```python
from build123d import *

# Parameters (mm, degrees)
SKETCH1_W           = 318
SKETCH1_H           = 8
BOSS_EXTRUDE1_DEPTH = 4.8
BOSS_EXTRUDE2_DEPTH = 0.79375
BOSS_EXTRUDE3_DEPTH = 0.79375
BOSS_EXTRUDE4_DEPTH = 0.79375
FILLET1_R           = 2.5


with BuildPart() as part:
    # Sketch1 → Boss-Extrude1 (new, symmetric)
    with BuildSketch(Plane.XY):
        Rectangle(SKETCH1_W, SKETCH1_H)
    extrude(amount=BOSS_EXTRUDE1_DEPTH, both=True)

    # Sketch3 → Boss-Extrude2 (add, symmetric)
    with BuildSketch(Plane.XY):
        Polygon((-64, 0), (-46.939710612, 195), (16.260289388, 195), (16, 0), align=None)
    boss_extrude2 = extrude(amount=BOSS_EXTRUDE2_DEPTH, both=True)

    # Mirror1: Boss-Extrude2 across plane
    add(boss_extrude2.mirror(Plane.ZX))

    # Sketch6 → Boss-Extrude3 (add, symmetric)
    with BuildSketch(Plane(origin=(0, 0, 0), x_dir=(1, 0, 0), z_dir=(0, 1, 0))):
        Polygon((159, -4.8), (166.766007972, -74.8), (145.966007972, -74.8), (107, -4.8), align=None)
    extrude(amount=BOSS_EXTRUDE3_DEPTH, both=True)

    # Sketch8 → Boss-Extrude4 (add, symmetric)
    with BuildSketch(Plane.XY):
        Polygon((159, 0), (177.834948036, 85.2), (153.758948036, 85.2), (112.7, 0), align=None)
    boss_extrude4 = extrude(amount=BOSS_EXTRUDE4_DEPTH, both=True)

    # Mirror2: Boss-Extrude4 across plane
    add(boss_extrude4.mirror(Plane.ZX))

    # Fillet1
    fillet1_edges = [part.edges().sort_by_distance(p)[0] for p in [
        (-159, 0, 4.8),
        (-159, 0, -4.8),
    ]]
    fillet(fillet1_edges, radius=FILLET1_R)


solid = part.part
```
Could you check a few things on this model? Use its own coordinates, in mm. A direction names the side the tool comes from. Round coordinates to 2 decimals unless told otherwise and drop trailing zeros. Write each loop counter-clockwise with the first axis right and the second up, starting at its lowest first coordinate (ties: lowest second). Pieces come first, ordered by that corner, then holes. Notation, with made-up numbers: M -11,32.5 L 5,32.5 A17 cw 5,36.5 Z; hole C 21,2.5 d9. An arc over 180 degrees is marked long. Answer in a Markdown table with one row per item. Add a question column.
Q1. Will these pins go through, and if not, where does the flat tip stop? pin 1 Ø24 at (x, y) = (-13.5, -86.5) entering from +Z; pin 2 Ø5 at (x, z) = (-28, 2) entering from +Y; pin 3 Ø19 at (x, y) = (132, -60.5) entering from -Z; pin 4 Ø8 at (x, z) = (103, 5) entering from +Y.
Q2. Imagine slicing it at C-C (z = 66.5). Please give me the cut outline in (x, y).
Q3. Imagine slicing it at A-A (y = 27). Please give me the cut outline in (x, z), then the cut area to 3 significant figures.
Q4. If I drill on line 1 (Y direction, x = 145, z = 32); line 2 (X direction, y = -1, z = 2), over which ranges is the centre line in solid material (lowest first)? Write a range as from..to.
Q5. Imagine slicing it at D-D (y = -23.5). Please give me the cut outline in (x, z).
Q6. If we mould it in two halves opening along X, with no side actions, what happens to faces 1 (the flat face through (134.47, 45.17, 0.01)), 2 (the flat face through (168.286, -42.004, 0.011)), 3 (the flat face through (-23, 101, -0.794))? For each: +X half, -X half, draft (parallel to the pull), parting line (faces both ways), or undercut.
Q7. Imagine slicing it at B-B (x = -19). Please give me the cut outline in (y, z), then the cut area to 3 significant figures.
Q8. On a 3-axis mill with a long thin cutter (end or side, diameter ignored), from which of +Z, -Z, +X, -X, +Y, -Y can I reach the whole of each face in a straight line? I mean faces 4 (the flat face through (-55.412, -98.163, 0.011)), 5 (the flat face through (144, -0.794, 32)), 6 (the flat face through (134.47, -45.17, 0.01)), 7 (the flat face through (-23, 101, 0.794)), 8 (the flat face through (-23, -101, -0.794)). Say none if no direction works.
Values:
| question | item | result |
|---|---|---|
| 1 | pin 1 | z = 0.79 |
| 1 | pin 2 | y = 195 |
| 1 | pin 3 | z = -0.79 |
| 1 | pin 4 | y = 4 |
| 2 | outline | M 141.35,-0.79 L 165.85,-0.79 L 165.85,0.79 L 141.35,0.79 Z |
| 3 | outline | M -61.64,-0.79 L 16.04,-0.79 L 16.04,0.79 L -61.64,0.79 Z; M 125.71,-0.79 L 164.97,-0.79 L 164.97,0.79 L 125.71,0.79 Z |
| 3 | area | 186 mm^2 |
| 4 | line 1 | -0.79..0.79 |
| 4 | line 2 | -159..159 |
| 5 | outline | M -61.94,-0.79 L 16.03,-0.79 L 16.03,0.79 L -61.94,0.79 Z; M 124.02,-0.79 L 164.2,-0.79 L 164.2,0.79 L 124.02,0.79 Z |
| 6 | face 1 | undercut |
| 6 | face 2 | +X half |
| 6 | face 3 | draft |
| 7 | outline | M -195,-0.79 L -4,-0.79 L -4,-4.8 L 4,-4.8 L 4,-0.79 L 195,-0.79 L 195,0.79 L 4,0.79 L 4,4.8 L -4,4.8 L -4,0.79 L -195,0.79 Z |
| 7 | area | 683 mm^2 |
| 8 | face 4 | +Z, -Z, -X, -Y |
| 8 | face 5 | +Z, +X, -X, -Y |
| 8 | face 6 | +Z, -Z, -Y |
| 8 | face 7 | +Z, +X, -X, +Y |
| 8 | face 8 | -Z, +X, -X, -Y |
